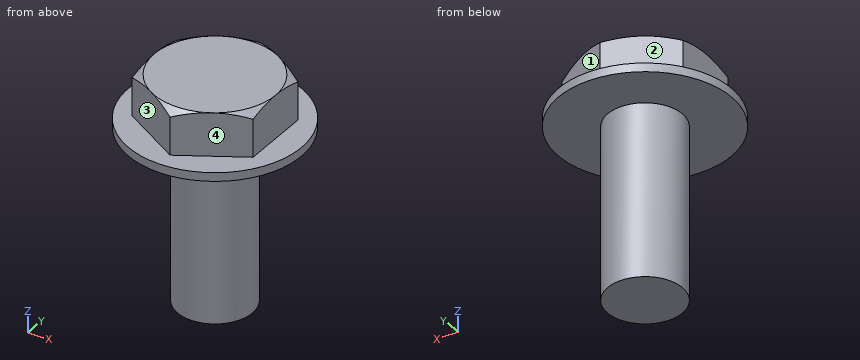
Solid Edge part; units mm, degrees
sketch "Sketch1" plane through (0, 0, 0) normal (0, 0, 1) x (1, 0, 0)
  line L0 (-3.5, -2.0207) -> (0, -4.0415)
  line L1 (0, -4.0415) -> (3.5, -2.0207)
  line L2 (3.5, -2.0207) -> (3.5, 2.0207)
  line L3 (3.5, 2.0207) -> (0, 4.0415)
  line L4 (0, 4.0415) -> (-3.5, 2.0207)
  line L5 (-3.5, 2.0207) -> (-3.5, -2.0207)
extrude "Protrusion1" add sketch "Sketch1" against normal blind 2.5
sketch "Sketch2" plane through (0, 0, 0) normal (0, -1, 0) x (1, 0, 0)
  line L0 (5.4053, -1.1) -> (5.2199, 0)
  line L1 (5.2199, 0) -> (3.5, 0)
  line L2 (3.5, 0) -> (5.4053, -1.1)
revolve "RevolvedCutout1" cut sketch "Sketch2" angle 360 about axis through (0, 0, 0) along (0, 0, 1)
sketch "Sketch3" plane through (0, 0, -2.5) normal (0, 0, -1) x (0.866, 0.5, 0)
  circle A0 centre (0, 0) radius 5
extrude "ExtrudedProtrusion_3" add sketch "Sketch3" along normal blind 0.5
sketch "Sketch4" plane through (0, 0, -3) normal (0, 0, -1) x (1, 0, 0)
  circle A0 centre (0, 0) radius 2.16
extrude "ExtrudedProtrusion_4" add sketch "Sketch4" along normal blind 10
Build history of the part. All positions in model axes, mm. Face numbers are marked on the shaded views. A direction names the side the tool comes from. Give positions to 0.01 mm unless a question says otherwise; leave off trailing zeros. Order: outer loops, then holes, each group sorted by start corner. A loop starts at its lowest first (then second) coordinate and runs counter-clockwise, first axis right, second up. Notation, with made-up numbers: M 60.25,-14.75 L 112.25,-14.75 A4 cw 112.25,-10.75 Z; hole C 34,87.5 d5. An arc over 180 degrees is marked long. Return JSON: item names as keys, results as strings.
Q1. Band-saw the part on B-B (y = -4.5). Give the cut face in (x, z).
Answer list:
{"outline": "M -2.18,-3 L 2.18,-3 L 2.18,-2.5 L -2.18,-2.5 Z"}
Q2. Wall check: probe 1 along Y at (x, z) = (0, -5.75); probe 2 along Z at (x, y) = (-4.5, -0.5); probe 3 along Z at (x, y) = (-2.75, -0.5). Give the ranges that are in metal, low to high. Write a range as from..to.
Answer list:
{"probe 1": "y = -2.16..2.16", "probe 2": "z = -3..-2.5", "probe 3": "z = -3..0"}
Q3. 3-axis set-ups, long thin cutter, end or side, ignore diameter. For the marked faces 1, 2, 3 and 4: which of +Z, -Z, +X, -X, +Y, -Y reach the whole face in a straight line?
Answer list:
{"face 1": "+Z, +X, +Y", "face 2": "+Z, -X, +Y", "face 3": "+Z, -X, -Y", "face 4": "+Z, +X, -Y"}
Q4. Band-saw the part on A-A (x = 4). Give the cut face in (y, z), then the cut area to 3 significant figures.
Answer list:
{"outline": "M -3,-3 L 3,-3 L 3,-2.5 L -3,-2.5 Z", "area": "3.00 mm^2"}
Q5. Flat gauge pins, fed straight in: pin 1 (0.8 mm diameter, centred on y = 0, z = -1, fed in from +X); pin 2 (1 mm diameter, centred on x = 1, y = -3, fed in from -Z); pin 3 (3 mm diameter, centred on y = -1, z = -11.5, fed in from +X); pin 4 (3 mm diameter, centred on y = -0.5, z = -1.5, fed in from -X). Where does each tip first touch, or does it go through?
Answer list:
{"pin 1": "stops at x = 3.5", "pin 2": "stops at z = -3", "pin 3": "stops at x = 2.16", "pin 4": "stops at x = -5"}
Q6. Band-saw the part on C-C (z = -10). Give the cut face in (x, y).
Answer list:
{"outline": "C 0,0 d4.32"}
